Autodesk Inventor part; units mm, degrees
ref_plane "YZ Plane" through (0, 0, 0) normal (1, 0, 0) x (0, 1, 0)
ref_plane "XZ Plane" through (0, 0, 0) normal (0, 1, 0) x (-1, 0, 0)
ref_plane "XY Plane" through (0, 0, 0) normal (0, 0, 1) x (1, 0, 0)
sketch "Sketch1" plane through (0, 0, 0) normal (0, 0, 1) x (1, 0, 0)
  arc A0 (34.6858, 43.8208) -> (31.9926, 43.8208) centre (33.3392, 24.5638) ccw
  circle A1 centre (33.3392, 24.5638) radius 20.066
  circle A2 centre (33.3392, 24.5638) radius 22.606
  line L0 (34.6858, 43.8208) -> (34.739, 44.581)
  line L1 (31.9926, 43.8208) -> (31.9395, 44.581)
  point P0 (0, 0)
  dimension "d0" = 38.608
  dimension "d3" = 0.762
  dimension "d4" = 2.54
extrude "Extrusion2" add sketch "Sketch1" along normal mid plane 14.478
extrude "Extrusion3" add sketch "Sketch1" along normal mid plane 13.97 contours A0 L1 A1 L0 picked at (34.4103, 44.3421)
pattern_circular "Circular Pattern1" count 15 over 360 about axis through (33.3392, 24.5638, 0) along (0, 0, 1) of "Extrusion3"
properties part number "Automoblox TireTL"
Build history of the part. All positions in model axes, mm. A direction names the side the tool comes from. Coordinates: 2 decimals unless noted, no trailing zeros. Order: outer loops, then holes, each group sorted by start corner. A loop starts at its lowest first (then second) coordinate and runs counter-clockwise, first axis right, second up. Notation, with made-up numbers: (57, 82) -> (112, 82) arc R13 cw to (112, 93) -> close; hole circle Ø10 at (-3, -27). An arc over 180 degrees is marked (long way). Answer in a Markdown table with one row per item. Add a question column.
Q1. Which spindle directions (+Z, -Z, +X, -X, +Y, -Y) get a long thin tool onto all of the face, cutting with end or side? Do faces 1 (the face through (41.3, 42.5, -6.985)), 2 (the face through (52, 31, 6.985)), 3 (the face through (51.69, 30.55, -0.1)). Say none if no direction does.
Q2. Drop flat-ended pins along their axis: pin 1 (1.4 mm diameter, centred on x = 42, y = 42.5, fed in from +Z); pin 2 (1.5 mm diameter, centred on x = 36, z = -4, fed in from -Y); pin 3 (2 mm diameter, centred on x = 34, z = 1.5, fed in from +Y); pin 4 (3 mm diameter, centred on y = 41.5, z = 4, fed in from +X). Give the stop position or say it passes through.
Q3. Band-saw the part on B-B, the plane x = 41.5. List the corners of the cut face in (y, z) (3 decimals).
Q4. Wall check: line 1 along X through (y, z) = (25, 3.5); line 2 along X through (y, z) = (16, -1.25); line 3 along Y through (x, z) = (34, -2.5). Give the ranges that are in metal, low to high. Write a range as [from, to].
Q5. Mould opens along X. For faces 4 (the face through (25, 6, 7.239)), 5 (the face through (29.34, 5.68, -0.1)), 6 (the face through (15.4, 38.32, -0.1)) say: +X half, -X half, draft (parallel to the pull), parting line (faces both ways), or undercut.
Q6. Band-saw the part on A-A, the plane y = 14.5. List the corners of the cut face in (x, z) (3 decimals).
Answers follow:
| question | item | result |
|---|---|---|
| 1 | face 1 | -Z |
| 1 | face 2 | +Z |
| 1 | face 3 | +Z, -Z |
| 2 | pin 1 | z = 7.24 |
| 2 | pin 2 | y = 2.04 |
| 2 | pin 3 | y = 47.17 |
| 2 | pin 4 | x = 49.85 |
| 3 | outline | (3.482, -7.239) -> (6.232, -7.239) -> (6.232, 7.239) -> (3.482, 7.239) -> close; (42.058, -6.985) -> (42.895, -6.985) -> (42.895, -7.239) -> (45.645, -7.239) -> (45.645, 7.239) -> (42.895, 7.239) -> (42.895, 6.985) -> (42.058, 6.985) -> close |
| 4 | line 1 | [10.74, 13.28], [53.4, 55.94] |
| 4 | line 2 | [12.42, 15.19], [15.78, 16.04], [50.64, 50.9], [51.49, 54.26] |
| 4 | line 3 | [1.97, 4.51], [43.86, 47.16] |
| 5 | face 4 | draft |
| 5 | face 5 | undercut |
| 5 | face 6 | parting line |
| 6 | outline | (13.097, -7.239) -> (15.979, -7.239) -> (15.979, -6.985) -> (16.866, -6.985) -> (16.866, 6.985) -> (15.979, 6.985) -> (15.979, 7.239) -> (13.097, 7.239) -> close; (49.812, -6.985) -> (50.699, -6.985) -> (50.699, -7.239) -> (53.582, -7.239) -> (53.582, 7.239) -> (50.699, 7.239) -> (50.699, 6.985) -> (49.812, 6.985) -> close |
